```python
from build123d import *

# Parameters (mm, degrees)
SKETCH1_R           = 6.24205
SKETCH1_R_2         = 3.175
BOSS_EXTRUDE1_DEPTH = 7.14502
CHAMFER1_SIZE       = 0.1905
CHAMFER2_SIZE       = 0.254
SKETCH3_W           = 2.0193
SKETCH3_H           = 6.24205


with BuildPart() as part:
    # Sketch1 → Boss-Extrude1 (new body)
    with BuildSketch(Plane(origin=(0, 0, 0), x_dir=(1, 0, 0), z_dir=(0, 1, 0))):
        with Locations(Location((0, 0, 0), (0, 0, 90))):
            Circle(SKETCH1_R)
        with Locations(Location((0, 0, 0), (0, 0, 90))):
            Circle(SKETCH1_R_2, mode=Mode.SUBTRACT)
    extrude(amount=BOSS_EXTRUDE1_DEPTH)

    # Chamfer1
    chamfer1_edges = [part.edges().sort_by_distance(p)[0] for p in [
        (0, 0, 6.24205),
        (0, 7.14502, 6.24205),
    ]]
    chamfer(chamfer1_edges, length=CHAMFER1_SIZE)

    # Chamfer2
    chamfer2_edges = [part.edges().sort_by_distance(p)[0] for p in [
        (0, 0, 3.175),
        (0, 7.14502, 3.175),
    ]]
    chamfer(chamfer2_edges, length=CHAMFER2_SIZE)

    # Sketch3 → #10-32 Tapped Hole1 (revolve, cut)
    with BuildSketch(Plane.ZX.offset(3.57251)):
        with Locations((1.00965, 3.121025)):
            Rectangle(SKETCH3_W, SKETCH3_H)
    revolve(axis=Axis((-6.35, 3.57251, 0), (1, 0, 0)), mode=Mode.SUBTRACT)


solid = part.part
```
CAD build for the part. Positions are in the model's coordinates, mm. A direction names the side the tool comes from. Round coordinates to 2 decimals unless told otherwise and drop trailing zeros. Order: outer loops, then holes, each group sorted by start corner. A loop starts at its lowest first (then second) coordinate and runs counter-clockwise, first axis right, second up. Notation, with made-up numbers: (72.5, -18) - (81.5, -18) arc R15 cw to (81.5, -8) - close; hole circle Ø5 at (-25.75, 37). An arc over 180 degrees is marked (long way). Answer as CSV lines item,"result". Start each with the question number.
1. Saw through at A-A, the plane z = 0. Count the separate pieces of the cut face and the enclosed holes in it, and give its area (3 significant figures).
2. Saw through at C-C, the plane y = 6.25. Write the cut outline in (x, z) (3 decimals).
3. Pin check, flat tips, straight feed: pin 1 (1 mm diameter, centred on y = 4, z = 3, fed in from +X); pin 2 (1.5 mm diameter, centred on x = -1.5, z = -1.5, fed in from -Y); pin 3 (1.5 mm diameter, centred on y = 5, z = 2.5, fed in from -X); pin 4 (2 mm diameter, centred on x = 2, y = 3, fed in from -Z). Stop position of each tip, or through.
4. Saw through at D-D, the plane y = 3. Write the cut outline in (x, z) (3 decimals).
5. Tool access for faces 1 (the face through (4.373, 2.966, 1.926)), 2 (the face through (3, 7.145, -3)): list every direction of +Z, -Z, +X, -X, +Y, -Y with a clear straight run to the whole face (end or side of a thin tool).
6. Drill centre lines: L1, parallel to Y at x = 4.95, z = 0; L2, parallel to Z at x = 0.75, y = 6; L3, parallel to X at y = 5.5, z = -2.75. Where is each one in solid material? Low to high. Write a range as [from, to].
7. Pull direction X, two halves, no side cores. Call faces 3 (the face through (-6.19, 3.53, 0.81)), 4 (the face through (-3.15, 3.53, 0.41)), 5 (the face through (3, 0, -3)): +X half, -X half, draft (parallel to the pull), parting line (faces both ways), or undercut.
Model answer:
1,separate pieces,"3"
1,enclosed holes,"0"
1,area,"31.2 mm²"
2,outline,"circle Ø12.484 at (0, 0); hole circle Ø6.35 at (0, 0)"
3,pin 1,"stops at x = 5.72"
3,pin 2,"passes through"
3,pin 3,"stops at x = -5.99"
3,pin 4,"stops at z = -6.16"
4,outline,"(2.516, -1.936) arc R3.175 cw (long way) to (2.516, 1.936) - (5.934, 1.936) arc R6.242 ccw (long way) to (5.934, -1.936) - close"
5,face 1,"+X"
5,face 2,"+Z, -Z, +X, -X, +Y"
6,L1,"y = [0, 1.55], [5.59, 7.15]"
6,L2,"z = [-6.2, -3.09], [3.09, 6.2]"
6,L3,"x = [-5.6, -1.59], [1.59, 5.6]"
7,face 3,"parting line"
7,face 4,"undercut"
7,face 5,"draft"
